from build123d import *

# Parameters (mm, degrees)
BOSS_EXTRUDE1_DEPTH = 2.032
FILLET1_R           = 2.54
SKETCH4_R           = 1.5875
CUT_EXTRUDE1_DEPTH  = 19.05
FILLET6_R           = 2.032
FILLET7_R           = 1.524


with BuildPart() as part:
    # Sketch1 → Boss-Extrude1 (new body)
    with BuildSketch(Plane(origin=(0, 0, 0), x_dir=(1, 0, 0), z_dir=(0, 1, 0))):
        with BuildLine():
            Line((-5.08, -7.62), (-5.08, -5.08))
            Line((-5.08, -5.08), (-7.62, -5.08))
            ThreePointArc((-7.62, -5.08), (-12.7, 0), (-7.62, 5.08))
            Line((-7.62, 5.08), (-5.08, 5.08))
            Line((-5.08, 5.08), (-5.08, 7.62))
            ThreePointArc((-5.08, 7.62), (0, 12.7), (5.08, 7.62))
            Line((5.08, 7.62), (5.08, 5.08))
            Line((5.08, 5.08), (7.62, 5.08))
            ThreePointArc((7.62, 5.08), (12.7, 0), (7.62, -5.08))
            Line((7.62, -5.08), (5.08, -5.08))
            Line((5.08, -5.08), (5.08, -7.62))
            ThreePointArc((5.08, -7.62), (0, -12.7), (-5.08, -7.62))
        make_face()
    extrude(amount=BOSS_EXTRUDE1_DEPTH)

    # Fillet1
    fillet1_edges = [part.edges().sort_by_distance(p)[0] for p in [
        (-5.08, 1.016, -5.08),
        (-5.08, 1.016, 5.08),
        (5.08, 1.016, 5.08),
        (5.08, 1.016, -5.08),
    ]]
    fillet(fillet1_edges, radius=FILLET1_R - 0.0001)  # a hair under: the kernel refuses the full size

    # Loft1: read off the stored shape, not the designer's step
    # Loft1: loft between two sections, ruled curve by curve
    loft1_from = [
        Edge.make_bspline([(6.165113119, 2.032, -1.52114438), (3.12282436, 2.032, -13.851370619), (-9.207401879, 2.032, -10.809081859), (-6.165113119, 2.032, 1.52114438), (-3.12282436, 2.032, 13.851370619), (9.207401879, 2.032, 10.809081859), (6.165113119, 2.032, -1.52114438)], [0, 0, 0, 0, 0.5, 0.5, 0.5, 1, 1, 1, 1], 3, [1, 0.333333333, 0.333333333, 1, 0.333333333, 0.333333333, 1]),
    ]
    loft1_to = [
        Edge.make_bspline([(2.787065251, 21.082, 1.520819611), (5.828704472, 21.082, -4.05331089), (0.254573971, 21.082, -7.094950112), (-2.787065251, 21.082, -1.520819611), (-5.828704472, 21.082, 4.05331089), (-0.254573971, 21.082, 7.094950112), (2.787065251, 21.082, 1.520819611)], [0, 0, 0, 0, 0.5, 0.5, 0.5, 1, 1, 1, 1], 3, [1, 0.333333333, 0.333333333, 1, 0.333333333, 0.333333333, 1]),
    ]
    loft1 = Solid(Shell([*[Face.make_surface_from_curves(loft1_from[k], loft1_to[k]) for k in range(1)], Face(Wire(loft1_from)), Face(Wire(loft1_to))]))
    add(loft1)

    # Sketch4 → Cut-Extrude1 (cut)
    with BuildSketch(Plane(origin=(0, 21.082, 0), x_dir=(1, 0, 0), z_dir=(0, 1, 0))):
        with Locations(Location((0, 0, 0), (0, 0, 270))):
            Circle(SKETCH4_R)
    extrude(amount=-CUT_EXTRUDE1_DEPTH, mode=Mode.SUBTRACT)

    # Fillet6
    fillet6_edges = [part.edges().sort_by_distance(p)[0] for p in [
        (-6.165113119, 2.032, 1.52114438),
    ]]
    fillet(fillet6_edges, radius=FILLET6_R)

    # Fillet7
    fillet7_edges = [part.edges().sort_by_distance(p)[0] for p in [
        (-2.787065251, 21.082, -1.520819611),
    ]]
    fillet(fillet7_edges, radius=FILLET7_R)


solid = part.part
Geometry check sheet. Reference: the model listing, model coordinates, mm. A direction names the side the tool comes from. Give positions to 0.01 mm unless a question says otherwise; leave off trailing zeros. Loops run counter-clockwise (first coordinate to the right, second up) from the corner with the lowest first, then second, coordinate; pieces in that order, holes last.
(1) Thickness scan on L1, parallel to Y at x = -8.5, z = 3.5; L2, parallel to X at y = 3, z = -0.25; L3, parallel to X at y = 11.75, z = 0. Record the ranges inside material, lowest first.
From the geometry:
L1: y = 0 to 2.03
L2: x = -6.27 to -1.57, 1.57 to 6.27
L3: x = -4.44 to -1.59, 1.59 to 4.44
(2) Section check B-B on x = 8.75. Record the cut outline in (y, z), then the cut area to 3 significant figures.
From the geometry:
outline: (0, -4.95) - (2.03, -4.95) - (2.03, 4.95) - (0, 4.95) - close
area: 20.1 mm2
(3) Depth check by flat-ended pin: pin 1 Ø10 at (y, z) = (6.5, 2) entering from +X; pin 2 Ø2 at (y, z) = (12, 1) entering from -X; pin 3 Ø2 at (y, z) = (11.5, -2.5) entering from -X; pin 4 Ø12 at (y, z) = (17, -10) entering from -X. Enter the tip coordinate at first touch or a pass-through.
From the geometry:
pin 1: stops at x = 12.7
pin 2: stops at x = -4.52
pin 3: stops at x = -4.27
pin 4: passes through
(4) Section check A-A on z = 9.75. Record the cut outline in (x, y).
From the geometry:
outline: (-4.61, 0) - (4.61, 0) - (4.61, 2.03) - (-4.61, 2.03) - close
(5) Set-up check for faces 4 (the cylindrical face through (5.804, 1.03, -5.844)), 5 (the flat face through (0, 2.032, 0)): record each of +Z, -Z, +X, -X, +Y, -Y from which the full face is reachable in a straight line by a thin tool's end or side.
From the geometry:
face 4: -Z, +X, +Y, -Y
face 5: +Y
(6) Release check for a two-part mould opening along X. For faces 1 (the cylindrical face through (-0.966, 11.69, -1.26)), 2 (the cylindrical face through (-5.844, 1.03, -5.804)), 3 (the cylindrical face through (5.844, 1.03, 5.804)) record: released by +X, released by -X, zero draft, split by the parting line, or undercut.
From the geometry:
face 1: undercut
face 2: released by -X
face 3: released by +X
